Read the model definition and answer for the solid it produces. Units are mm, in the model's axes. A direction names the side the tool comes from. Give positions to 0.01 mm unless a question says otherwise; leave off trailing zeros. Order: outer loops, then holes, each group sorted by start corner. A loop starts at its lowest first (then second) coordinate and runs counter-clockwise, first axis right, second up. Notation, with made-up numbers: (54, 29) -> (72, 29) arc R33 cw to (72, 58) -> close; hole circle Ø11 at (34.5, -24.5). An arc over 180 degrees is marked (long way). Answer as CSV lines item,"result". Start each with the question number.
1) Find section A-A (x = -23). Determine the outline of the cut face in (y, z) (1 decimal).
2) Find section D-D (x = -44). Determine the outline of the cut face in (y, z) (1 decimal), and give its area (3 significant figures).
3) Flat-ended cylindrical pins translate along their axes: pin 1 Ø5.5 at (y, z) = (-7.5, -18.5) entering from +X; pin 2 Ø0.6 at (y, z) = (-11.5, -7) entering from -X; pin 3 Ø4.5 at (x, z) = (63.5, 12.5) entering from -Y (3 decimals). Find the tip coordinate at first contact, or state that the pin passes through.
4) Straight lines are drawn through the part: L1, parallel to Z at x = -6, y = -4.75; L2, parallel to X at y = -11, z = -19; L3, parallel to X at y = -10.5, z = 5 (3 decimals). For each, find the intervals that lie inside material, in ascending order. Write a range as from..to.
5) For faces 1 (the face through (-52.33, -15.7, 6.67)), 2 (the face through (41.275, -5, -38)), 3 (the face through (41.275, -5, 0)), determine the directions among +Z, -Z, +X, -X, +Y, -Y from which every point of the face is accessible in a straight line to the end or side of a thin tool.
6) Find section B-B (y = -6). Determine the outline of the cut face in (x, z) (1 decimal).
```python
from build123d import *

# Parameters (mm, degrees)
F0_W     = 101.6
F0_H     = 101.6
F0_W_2   = 82.55
F0_H_2   = 50.419
F1_DEPTH = 10.795
F2_W     = 101.6
F2_H     = 29.6545
F2_W_2   = 82.55
F2_H_2   = 19.05
F3_DEPTH = 6.35
F4_W     = 10.16
F4_H     = 101.6
F5_DEPTH = 22.86
F6_W     = 9.144
F6_H     = 101.6
F6_R     = 2.286
F7_DEPTH = 6.35
F8_R     = 5.08
F9_R     = 5.07999


# Not quite as in the source:
# - a fillet or chamfer is up to 0.001 mm smaller than in the source, because OpenCascade refuses the exact size


with BuildPart() as f1:
    # F0 (on Front) → F1 (new body)
    with BuildSketch(Plane.XZ):
        with Locations((0, -6.1595)):
            Rectangle(F0_W, F0_H)
        Polygon((-41.275, -29.0195), (0, -29.0195), (41.275, -29.0195), (41.275, -48.0695), (-41.275, -48.0695), align=None, mode=Mode.SUBTRACT)
        Rectangle(F0_W_2, F0_H_2, mode=Mode.SUBTRACT)
    extrude(amount=F1_DEPTH)

    # F2 (on face) → F3 (join)
    with BuildSketch(Plane.XZ.offset(10.795)):
        with Locations((0, -42.13225)):
            Rectangle(F2_W, F2_H)
        with Locations((0, -38.5445)):
            Rectangle(F2_W_2, F2_H_2, mode=Mode.SUBTRACT)
        with Locations((0, -38.5445)):
            Rectangle(F2_W_2, F2_H_2)
    extrude(amount=F3_DEPTH)

    # F4 (on face) → F5 (join)
    with BuildSketch(Plane.XZ.offset(17.145)):
        with Locations((-55.88, -6.1595)):
            Rectangle(F4_W, F4_H)
        with Locations((55.88, -6.1595)):
            Rectangle(F4_W, F4_H)
    extrude(amount=-F5_DEPTH)

    # F6 (on face) → F7 (join)
    with BuildSketch(Plane(origin=(0, 5.715, 0), x_dir=(-1, 0, 0), z_dir=(0, 1, 0))):
        with Locations((-65.532, -6.1595)):
            Rectangle(F6_W, F6_H)
        with Locations((-65.532, -44.2595)):
            Circle(F6_R, mode=Mode.SUBTRACT)
        with Locations((-65.532, 31.9405)):
            Circle(F6_R, mode=Mode.SUBTRACT)
        with Locations((65.532, -6.1595)):
            Rectangle(F6_W, F6_H)
        with Locations((65.532, -44.2595)):
            Circle(F6_R, mode=Mode.SUBTRACT)
        with Locations((65.532, 31.9405)):
            Circle(F6_R, mode=Mode.SUBTRACT)
    extrude(amount=-F7_DEPTH)

    # F8
    f8_edges = [f1.edges().sort_by_distance(p)[0] for p in [
        (-60.96, -17.145, -6.1595),
        (0, -17.145, -56.9595),
        (60.96, -17.145, -6.1595),
    ]]
    fillet(f8_edges, radius=F8_R)

    # F9 (radius 5.08 in the source; OpenCascade refuses exactly that, so slightly less here)
    f9_edges = [f1.edges().sort_by_distance(p)[0] for p in [
        (-50.8, -17.145, 8.66775),
        (0, -17.145, -27.305),
        (50.8, -17.145, 8.66775),
    ]]
    fillet(f9_edges, radius=F9_R)


solid = f1.part
```
Findings below:
1,outline,"(-17.1, -51.9) arc R5.1 ccw to (-12.1, -57) -> (0, -57) -> (0, -48.1) -> (-10.8, -48.1) -> (-10.8, -29) -> (0, -29) -> (0, -25.2) -> (-10.8, -25.2) -> (-10.8, -27.3) -> (-12.1, -27.3) arc R5.1 ccw to (-17.1, -32.4) -> close; (-10.8, 25.2) -> (0, 25.2) -> (0, 44.6) -> (-10.8, 44.6) -> close"
2,outline,"(-17.1, -51.9) arc R5.1 ccw to (-12.1, -57) -> (0, -57) -> (0, 44.6) -> (-10.8, 44.6) -> (-10.8, -27.3) -> (-12.1, -27.3) arc R5.1 ccw to (-17.1, -32.4) -> close"
2,area,"1,270 mm²"
3,pin 1,"x = 60.96"
3,pin 2,"x = -60.96"
3,pin 3,"y = -0.635"
4,L1,"-56.96..-48.07, -29.02..-25.21, 25.21..44.64"
4,L2,"-60.96..-50.8, 50.8..60.96"
4,L3,"-60.96..-41.275, 41.275..60.96"
5,face 1,"+Z, -Y"
5,face 2,"+Y"
5,face 3,"+Y, -Y"
6,outline,"(-61, -57) -> (61, -57) -> (61, 44.6) -> (-61, 44.6) -> close; hole (-41.3, -48.1) -> (41.3, -48.1) -> (41.3, -29) -> (-41.3, -29) -> close; hole (-41.3, -25.2) -> (41.3, -25.2) -> (41.3, 25.2) -> (-41.3, 25.2) -> close"
